Input: part model. Units: mm. Frame: model coordinates. A direction names the side the tool comes from. Round coordinates to 2 decimals unless told otherwise and drop trailing zeros. Order: outer loops, then holes, each group sorted by start corner. A loop starts at its lowest first (then second) coordinate and runs counter-clockwise, first axis right, second up. Notation, with made-up numbers: (29.5, 68) -> (33.5, 68) arc R28 cw to (33.5, 97) -> close; hole circle Ø9 at (-29, -0.75). An arc over 180 degrees is marked (long way). Use a Markdown table: item, result.
from build123d import *

# Parameters (mm, degrees)
BOSS_EXTRUDE1_DEPTH = 450
SKETCH3_R           = 2.25
CUT_EXTRUDE2_DEPTH  = 451.943333469


with BuildPart() as part:
    # Sketch1 → Boss-Extrude1 (new body)
    with BuildSketch(Plane.XY):
        with BuildLine():
            Line((-15.8, 0), (15.8, 0))
            Line((15.8, 0), (15.8, 4))
            Line((15.8, 4), (6.689237738, 4))
            Line((6.689237738, 4), (6.689237738, 8))
            Line((6.689237738, 8), (3.22379765, 13.439651325))
            ThreePointArc((3.22379765, 13.439651325), (0, 24.5), (-3.22379765, 13.439651325))
            Line((-3.22379765, 13.439651325), (-6.689237738, 8))
            Line((-6.689237738, 8), (-6.689237738, 4))
            Line((-6.689237738, 4), (-15.8, 4))
            Line((-15.8, 4), (-15.8, 0))
        make_face()
    extrude(amount=BOSS_EXTRUDE1_DEPTH)

    # Sketch3 → Cut-Extrude2 (cut, through all)
    with BuildSketch(Plane(origin=(0, 0, 0), x_dir=(1, 0, 0), z_dir=(0, 1, 0))):
        with Locations(Location((-11.244618869, -25, 0), (0, 0, 90))):
            Circle(SKETCH3_R)
        with Locations(Location((11.244618869, -25, 0), (0, 0, 90))):
            Circle(SKETCH3_R)
        with Locations(Location((-11.244618869, -125, 0), (0, 0, 90))):
            Circle(SKETCH3_R)
        with Locations(Location((11.244618869, -125, 0), (0, 0, 90))):
            Circle(SKETCH3_R)
        with Locations(Location((-11.244618869, -225, 0), (0, 0, 90))):
            Circle(SKETCH3_R)
        with Locations(Location((11.244618869, -225, 0), (0, 0, 90))):
            Circle(SKETCH3_R)
        with Locations(Location((-11.244618869, -325, 0), (0, 0, 90))):
            Circle(SKETCH3_R)
        with Locations(Location((11.244618869, -325, 0), (0, 0, 90))):
            Circle(SKETCH3_R)
        with Locations(Location((-11.244618869, -425, 0), (0, 0, 90))):
            Circle(SKETCH3_R)
        with Locations(Location((11.244618869, -425, 0), (0, 0, 90))):
            Circle(SKETCH3_R)
    extrude(amount=CUT_EXTRUDE2_DEPTH, mode=Mode.SUBTRACT)


solid = part.part
1) Cut plane A-A on z = 202.5. Return loops of the section in (x, y), and give its area (3 significant figures).
Results found:
| item | result |
|---|---|
| outline | (-15.8, 0) -> (15.8, 0) -> (15.8, 4) -> (6.69, 4) -> (6.69, 8) -> (3.22, 13.44) arc R6 ccw (long way) to (-3.22, 13.44) -> (-6.69, 8) -> (-6.69, 4) -> (-15.8, 4) -> close |
| area | 343 mm² |
2) Pull-direction query (Y, two-part tool) for faces 1 (the flat face through (0, 10, 0)), 2 (the flat face through (0, 0, 222)), 3 (the cylindrical face through (0.216, 24.496, 221.85)), 4 (the flat face through (-11, 4, 222)); classes: +Y half, -Y half, draft (parallel to the pull), parting line (faces both ways), or undercut.
Results found:
| item | result |
|---|---|
| face 1 | draft |
| face 2 | -Y half |
| face 3 | undercut |
| face 4 | +Y half |
3) Set-up query: faces 5 (the flat face through (11, 4, 222)), 6 (the flat face through (0, 10, 450)). Return all of +Z, -Z, +X, -X, +Y, -Y with unobstructed straight access to the full face (end or side cutting, diameter ignored); none if empty.
Results found:
| item | result |
|---|---|
| face 5 | +Z, -Z, +X, +Y |
| face 6 | +Z, +X, -X, +Y, -Y |
4) Line query: L1, parallel to X at y = 2.5, z = 225; L2, parallel to Z at x = -11, y = 2; L3, parallel to Y at x = -1, z = 423. Output: solid intervals per line, ascending. Write a range as [from, to].
Results found:
| item | result |
|---|---|
| L1 | x = [-15.8, -13.49], [-8.99, 8.99], [13.49, 15.8] |
| L2 | z = [0, 22.76], [27.24, 122.76], [127.24, 222.76], [227.24, 322.76], [327.24, 422.76], [427.24, 450] |
| L3 | y = [0, 24.42] |
5) Pin query (flat end, axial travel): pin 1 Ø5 at (y, z) = (20.5, 279) entering from -X; pin 2 Ø4.5 at (y, z) = (7, 331.5) entering from +X; pin 3 Ø6 at (x, z) = (11.24, 225) entering from +Y; pin 4 Ø4 at (x, z) = (11.24, 325) entering from -Y. Return the tip coordinate at first contact, or that it passes through.
Results found:
| item | result |
|---|---|
| pin 1 | stops at x = -6 |
| pin 2 | stops at x = 6.69 |
| pin 3 | stops at y = 4 |
| pin 4 | passes through |
